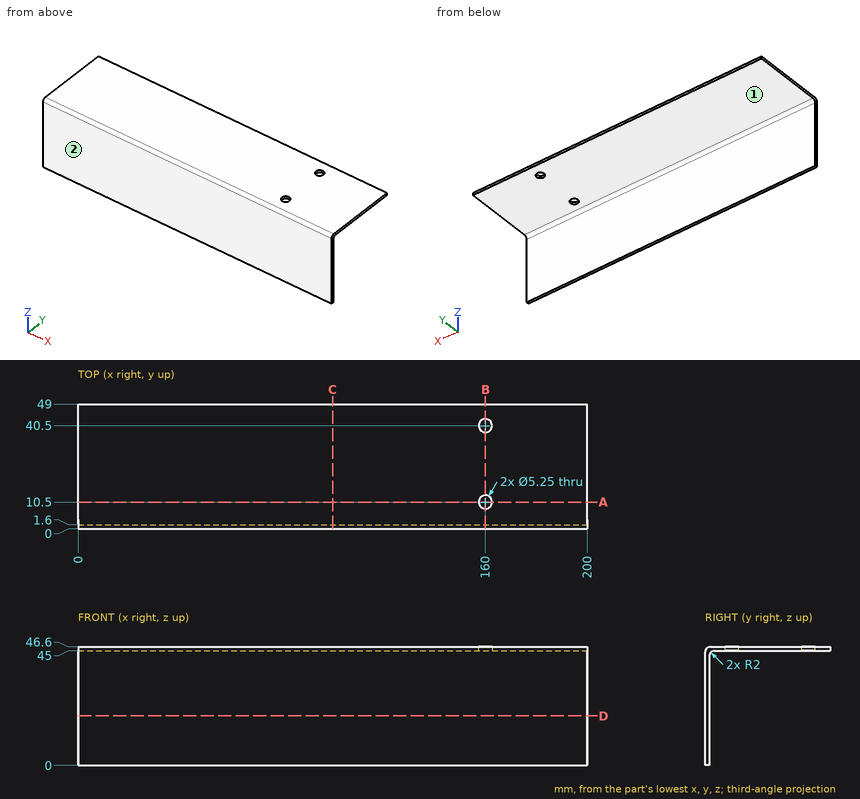
Here's the drawing with two shaded views (mm, measured from the low corner). I have some questions. A direction names the side the tool comes from. Coordinates: 2 decimals unless noted, no trailing zeros. Loops run counter-clockwise (first coordinate to the right, second up) from the corner with the lowest first, then second, coordinate; pieces in that order, holes last. Notation, with made-up numbers: M 13,-40 L 71,-40 A10 cw 71,-31 Z; hole C -4,31.5 d3. An arc over 180 degrees is marked long. Put each result on its own line as item: value. Start each with the question number.
(1) Imagine slicing it at A-A on y = 10.5. List the corners of the cut face in (x, z) for me (3 decimals), and give its area (3 significant figures).
(2) Imagine slicing it at C-C on x = 100. List the corners of the cut face in (y, z) for me.
(3) Imagine slicing it at D-D on z = 19.5. List the corners of the cut face in (x, y) for me, and give its area (3 significant figures).
(4) I need wall thicknesses on probe 1 along Y at (x, z) = (160, 46) (3 decimals); probe 2 along Y at (x, z) = (160, 45.8) (3 decimals); probe 3 along Z at (x, y) = (156, 7.5). Which ranges of each line are inside material? Lowest first, please.
(5) Will these pins go through, and if not, where does the flat tip stop? pin 1 Ø13 at (x, z) = (111, 28) entering from +Y; pin 2 Ø5 at (x, y) = (51, 7) entering from -Z.
(6) Imagine slicing it at B-B on x = 160. List the corners of the cut face in (y, z) for me (3 decimals).
(7) Which directions (+Z, -Z, +X, -X, +Y, -Y) give clear straight access to the entire face, cutting with the end or side of a thin tool? Please do the marked faces 1 and 2.
Worked answers:
1. outline: M 0,45 L 157.375,45 L 157.375,46.6 L 0,46.6 Z; M 162.625,45 L 200,45 L 200,46.6 L 162.625,46.6 Z
1. area: 312 mm2
2. outline: M 0,0 L 1.6,0 L 1.6,43 A2 cw 3.6,45 L 49,45 L 49,46.6 L 2,46.6 A2 ccw 0,44.6 Z
3. outline: M 0,0 L 200,0 L 200,1.6 L 0,1.6 Z
3. area: 320 mm2
4. probe 1: y = 0.572 to 7.875, 13.125 to 37.875, 43.125 to 49
4. probe 2: y = 0.4 to 7.875, 13.125 to 37.875, 43.125 to 49
4. probe 3: z = 45 to 46.6
5. pin 1: stops at y = 1.6
5. pin 2: stops at z = 45
6. outline: M 0,0 L 1.6,0 L 1.6,43 A2 cw 3.6,45 L 7.875,45 L 7.875,46.6 L 2,46.6 A2 ccw 0,44.6 Z; M 13.125,45 L 37.875,45 L 37.875,46.6 L 13.125,46.6 Z; M 43.125,45 L 49,45 L 49,46.6 L 43.125,46.6 Z
7. face 1: -Z, +X, -X, +Y
7. face 2: +Z, -Z, +X, -X, -Y
